Read the model definition and answer for the solid it produces. Units are mm, in the model's axes. A direction names the side the tool comes from. Coordinates: 2 decimals unless noted, no trailing zeros. Loops run counter-clockwise (first coordinate to the right, second up) from the corner with the lowest first, then second, coordinate; pieces in that order, holes last. Notation, with made-up numbers: (67, 83) - (122, 83) arc R18 cw to (122, 97) - close; hole circle Ø1 at (25, 48). An arc over 180 degrees is marked (long way). Use one line per item in the form item = value.
from build123d import *

# Parameters (mm, degrees)
F0_W            = 120
F0_H            = 2.25
F0_H_2          = 6.5
F1_DEPTH        = 2.5
F2_DEPTH        = 6
F6_D            = 3
F6_CSINK_D      = 5
F6_CSINK_ANGLE  = 90
F7_D            = 2.5
F8_D            = 3.5
F8_DEPTH        = 3
F8_TIP          = 1.0515060833
F10_D           = 1.5
F10_CSINK_D     = 3
F10_CSINK_ANGLE = 90


# Not quite as in the source:
# - a feature names something its author has since deleted; it is built from what else it names


with BuildPart() as f1:
    # F0 (on Top) → F1 (new body)
    with BuildSketch(Plane.XY):
        with Locations((0, 4.375)):
            Rectangle(F0_W, F0_H)
        Rectangle(F0_W, F0_H_2)
        with Locations((0, -4.375)):
            Rectangle(F0_W, F0_H)
    extrude(amount=F1_DEPTH)

    # F0 (on Top) → F2 (join)
    with BuildSketch(Plane.XY):
        with Locations((0, 4.375)):
            Rectangle(F0_W, F0_H)
        with Locations((0, -4.375)):
            Rectangle(F0_W, F0_H)
    extrude(amount=-F2_DEPTH)

    # F6 (through all)
    with Locations(Plane(origin=(0, 0, 0), x_dir=(1, 0, 0), z_dir=(0, 0, -1))):
        with Locations((-52.377641201, 0), (51.710255444, 0)):
            CounterSinkHole(F6_D / 2, F6_CSINK_D / 2, counter_sink_angle=F6_CSINK_ANGLE)

    # F7 (through all)
    with Locations(Plane(origin=(0, 0, 0), x_dir=(1, 0, 0), z_dir=(0, 0, -1))):
        with Locations((0, 0)):
            Hole(F7_D / 2)

    # F8
    with Locations(Plane.XZ.offset(5.5)):
        with Locations((-45, -4.5), (-35, -4.5), (-25, -4.5), (25, -4.5), (35, -4.5), (45, -4.5)):
            Hole(F8_D / 2, depth=F8_DEPTH)
            with Locations((0, 0, -(F8_DEPTH + F8_TIP / 2))):  # 118° drill point
                Cone(0, F8_D / 2, F8_TIP, mode=Mode.SUBTRACT)

    # F10 (through all)
    with Locations(Plane.XZ.offset(5.5)):
        with Locations((0, -3.5449948628)):
            CounterSinkHole(F10_D / 2, F10_CSINK_D / 2, counter_sink_angle=F10_CSINK_ANGLE)

    # F11: F1 across plane


with BuildPart() as f1_1:
    add(f1.part)
    add(f1.part.mirror(Plane.YZ))


solid = f1_1.part
Item 1: The part is cut by section A-A on x = 3. Give the vertices of the cut face in (y, z), plus the area to 3 significant figures.
Results below:
outline = (-5.5, -6) - (-3.25, -6) - (-3.25, 0) - (3.25, 0) - (3.25, -6) - (5.5, -6) - (5.5, 2.5) - (-5.5, 2.5) - close
area = 54.5 mm²
Item 2: Which of the six approach directions +Z, -Z, +X, -X, +Y, -Y give full straight-line access (tool end or side, diameter ignored) to faces 1 (the flat face through (-1, -3.25, -3)), 2 (the cylindrical face through (24.94, -4.36, -2.75)), 3 (the flat face through (-40, -4, -6)), 4 (the conical face through (-50.72, -0.03, 0.84))?
Results below:
face_1 = -Z, +X, -X
face_2 = -Y
face_3 = -Z, +X, -X, +Y, -Y
face_4 = -Z
Item 3: Find the intervals of material crossed by L1, parallel to Z at x = 0, y = -4.4 (3 decimals); L2, parallel to Y at x = 0, z = 1.25; L3, parallel to Y at x = 22.5, z = -1.75, in increasing order.
Results below:
L1 = -6 to -4.295, -2.795 to 2.5
L2 = -5.5 to -1.25, 1.25 to 5.5
L3 = -5.5 to -3.25, 3.25 to 5.5
Item 4: Each of these flat-tipped pins is pushed along its axis until it touches: P1, Ø1.7, axis at x = 0, z = -3.54, coming from the -Y side (3 decimals); P2, Ø0.9, axis at x = 0, z = -3.54, coming from the +Y side; P3, Ø2, axis at x = 5.5, y = -1, coming from the -Z side. Where does it stop, or does it pass through?
Results below:
P1 = -4.855
P2 = through
P3 = 0
Item 5: For a pull along X with two mould halves and no side action, classify faces 5 (the cylindrical face through (44.94, -4.36, -2.75)), 6 (the cylindrical face through (-25.06, -4.36, -2.75)), 7 (the flat face through (-53, -4, -6)) as +X half, -X half, draft (parallel to the pull), parting line (faces both ways), or undercut.
Results below:
face_5 = undercut
face_6 = undercut
face_7 = draft
